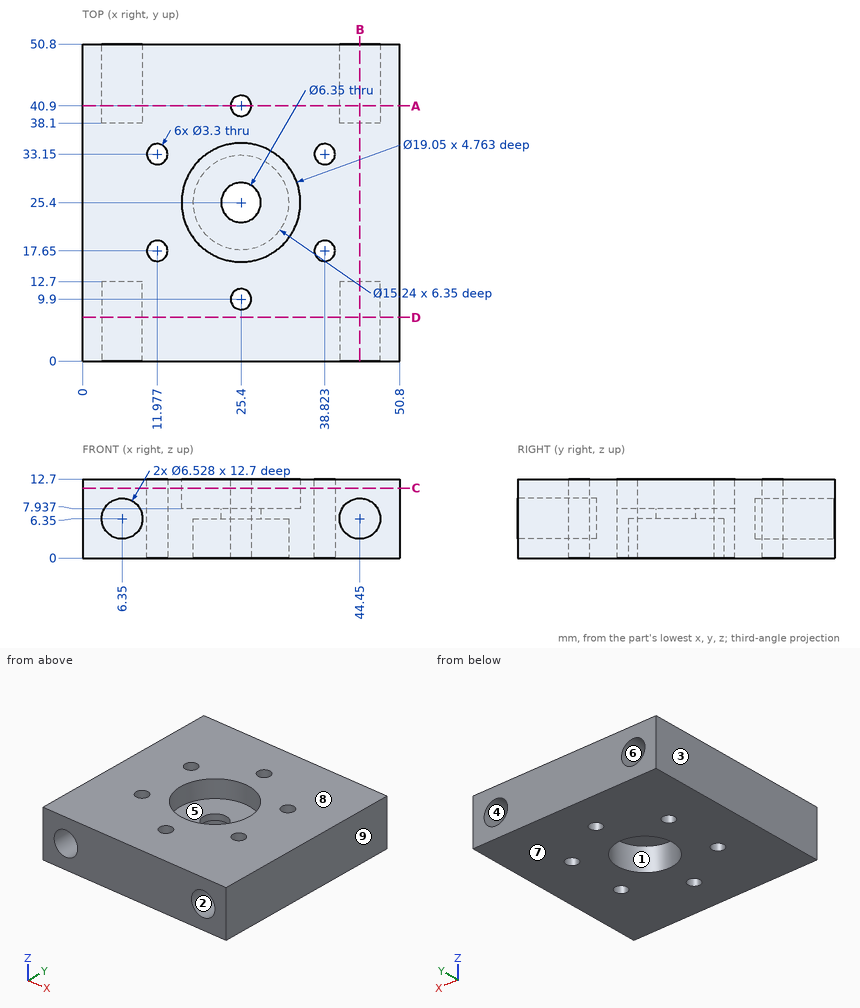
For this review, use the dimensioned drawing (mm, ordinates from the lowest corner) and the shaded views. A direction names the side the tool comes from. Give positions to 0.01 mm unless a question says otherwise; leave off trailing zeros. Order: outer loops, then holes, each group sorted by start corner. A loop starts at its lowest first (then second) coordinate and runs counter-clockwise, first axis right, second up. Notation, with made-up numbers: (21.25, 69.5) - (40.25, 69.5) arc R15 cw to (40.25, 76.5) - close; hole circle Ø1 at (14, -24). An arc over 180 degrees is marked (long way). Use a Markdown table: item, result. Add a question column.
(1) Add section D-D on y = 7. Give the boundary of the cut face in (x, z), then the cut area to 3 significant figures.
(2) Mouldability with a two-part tool opening along Z and no side actions: class the marked faces 6, 7, 8 and 9 as +Z half, -Z half, draft (parallel to the pull), parting line (faces both ways), or undercut.
(3) Wall thickness on probe 1 along X at (y, z) = (4, 6.35); probe 2 along X at (y, z) = (27, 9.5); probe 3 along Z at (x, y) = (44.45, 7): over which ranges is each line inside the solid? List them lowest first. Write a range as [from, to].
(4) Machinability: for the marked faces 1, 2, 3, 4 and 5, which of the approach directions +Z, -Z, +X, -X, +Y, -Y give a long, thin tool a straight path to every point of the face, cutting with its end or side? Answer none if there is none.
(5) Add section B-B on x = 44.45. Give the boundary of the cut face in (y, z).
(6) Clearance check with flat-ended pins moving along their axes: P1, Ø2, axis at x = 29, y = 18.5, coming from the +Z side; P2, Ø3, axis at x = 11.98, y = 17.65, coming from the -Z side. State where each tip first meets the part, or that it passes through.
(7) Add section C-C on z = 11.25. Give the number of separate pieces and of enclosed holes in the cut face, then the cut area to 3 significant figures.
(8) Add section A-A on y = 40.9. Give the boundary of the cut face in (x, z).
Report:
| question | item | result |
|---|---|---|
| 1 | outline | (0, 0) - (50.8, 0) - (50.8, 12.7) - (0, 12.7) - close; hole circle Ø6.53 at (6.35, 6.35); hole circle Ø6.53 at (44.45, 6.35) |
| 1 | area | 578 mm² |
| 2 | face 6 | undercut |
| 2 | face 7 | -Z half |
| 2 | face 8 | +Z half |
| 2 | face 9 | draft |
| 3 | probe 1 | x = [0, 3.09], [9.61, 41.19], [47.71, 50.8] |
| 3 | probe 2 | x = [0, 16.01], [34.79, 50.8] |
| 3 | probe 3 | z = [0, 3.09], [9.61, 12.7] |
| 4 | face 1 | -Z |
| 4 | face 2 | -Y |
| 4 | face 3 | +Z, -Z, -X, +Y, -Y |
| 4 | face 4 | +Y |
| 4 | face 5 | +Z |
| 5 | outline | (0, 0) - (50.8, 0) - (50.8, 3.09) - (38.1, 3.09) - (38.1, 9.61) - (50.8, 9.61) - (50.8, 12.7) - (0, 12.7) - (0, 9.61) - (12.7, 9.61) - (12.7, 3.09) - (0, 3.09) - close |
| 6 | P1 | stops at z = 7.94 |
| 6 | P2 | passes through |
| 7 | separate pieces | 1 |
| 7 | enclosed holes | 7 |
| 7 | area | 2,240 mm² |
| 8 | outline | (0, 0) - (23.75, 0) - (23.75, 12.7) - (0, 12.7) - close; (27.05, 0) - (50.8, 0) - (50.8, 12.7) - (27.05, 12.7) - close; hole circle Ø6.53 at (6.35, 6.35); hole circle Ø6.53 at (44.45, 6.35) |
